CAD build for the part. Positions are in the model's coordinates, mm. Face numbers are marked on the shaded views. A direction names the side the tool comes from. Coordinates: 2 decimals unless noted, no trailing zeros. Write each loop counter-clockwise with the first axis right and the second up, starting at its lowest first coordinate (ties: lowest second). Pieces come first, ordered by that corner, then holes. Notation, with made-up numbers: (-32, 85) - (24, 85) arc R26 ccw to (24, 106) - close; hole circle Ø4 at (54, 54). An arc over 180 degrees is marked (long way). One line per question, with ' | ' between items. Start each with the question number.
1. Which spindle directions (+Z, -Z, +X, -X, +Y, -Y) get a long thin tool onto all of the face, cutting with end or side? Do the marked faces 1, 2 and 3. Say none if no direction does.
2. Band-saw the part on A-A, the plane x = 33.5. Write the cut outline in (y, z), then the cut area to 3 significant figures.
3. Flat gauge pins, fed straight in: P1, Ø1.5, axis at x = -19, z = -2, coming from the +Y side; P2, Ø4, axis at x = 31, y = 9, coming from the +Z side; P3, Ø10, axis at y = 5, z = -8.5, coming from the -X side. Where does each tip first touch, or does it go through?
4. Two-plate mould, pull along Z, no slides. Class the marked faces 4, 5, 6 and 7: +Z half, -Z half, draft (parallel to the pull), parting line (faces both ways), or undercut.
5. Band-saw the part on D-D, the plane z = 14. Write the cut outline in (x, y), then the cut area to 3 significant figures.
6. Band-saw the part on C-C, the plane x = 16. Write the cut outline in (y, z), then the cut area to 3 significant figures.
7. Band-saw the part on B-B, the plane z = 0. Write the cut outline in (x, y), then the cut area to 3 significant figures.
8. Probe line 1 (Z direction, x = 43.5, y = 13); line 2 (Y direction, x = 27.5, z = 5); line 3 (Z direction, x = 9.5, y = 9.25). List the from-to ranges inside material, lowest first.
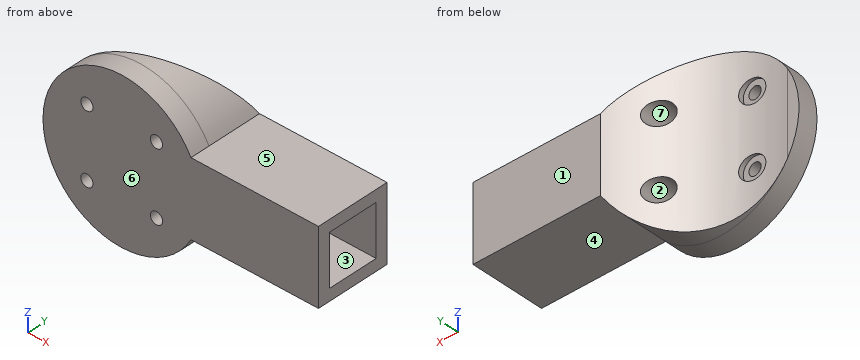
from build123d import *

# Parameters (mm, degrees)
BOSS_EXTRUDE1_DEPTH     = 2.5
SKETCH2_R               = 1.55
CUT_EXTRUDE1_DEPTH      = 2.5
SKETCH6_W               = 19
SKETCH6_H               = 19
BOSS_EXTRUDE3_DEPTH     = 32.400284093
SKETCH8_W               = 13
SKETCH8_H               = 13
CUT_EXTRUDE2_DEPTH      = 27.400284093
FILLET2_R               = 50
CUT_EXTRUDE4_REACH      = 57.642
CUT_EXTRUDE4_END_RADIUS = 50
SKETCH13_R              = 3


with BuildPart() as part:
    # Sketch1 → Boss-Extrude1 (new, symmetric)
    with BuildSketch(Plane(origin=(0, 0, 0), x_dir=(1, 0, 0), z_dir=(0, 1, 0))):
        with BuildLine():
            Line((17.599715907, 9.5), (50, 9.5))
            Line((50, 9.5), (50, -9.5))
            Line((50, -9.5), (17.599715907, -9.5))
            ThreePointArc((17.599715907, -9.5), (-20, 0), (17.599715907, 9.5))
        make_face()
    extrude(amount=BOSS_EXTRUDE1_DEPTH, both=True)

    # Sketch2 → Cut-Extrude1 (cut, symmetric)
    with BuildSketch(Plane(origin=(0, 0, 0), x_dir=(1, 0, 0), z_dir=(0, 1, 0))):
        with Locations(Location((8.838834765, 8.838834765, 0), (0, 0, 270))):
            Circle(SKETCH2_R)
        with Locations(Location((-8.838834765, 8.838834765, 0), (0, 0, 270))):
            Circle(SKETCH2_R)
        with Locations(Location((-8.838834765, -8.838834765, 0), (0, 0, 270))):
            Circle(SKETCH2_R)
        with Locations(Location((8.838834765, -8.838834765, 0), (0, 0, 270))):
            Circle(SKETCH2_R)
    extrude(amount=CUT_EXTRUDE1_DEPTH, both=True, mode=Mode.SUBTRACT)

    # Sketch6 → Boss-Extrude3 (add)
    with BuildSketch(Plane(origin=(50, 0, 0), x_dir=(0, 0, -1), z_dir=(1, 0, 0))):
        with Locations((0, 7)):
            Rectangle(SKETCH6_W, SKETCH6_H)
    extrude(amount=-BOSS_EXTRUDE3_DEPTH)

    # Sketch8 → Cut-Extrude2 (cut)
    with BuildSketch(Plane(origin=(50, 0, 0), x_dir=(0, 0, -1), z_dir=(1, 0, 0))):
        with Locations((0, 7)):
            Rectangle(SKETCH8_W, SKETCH8_H)
    extrude(amount=-CUT_EXTRUDE2_DEPTH, mode=Mode.SUBTRACT)

    # Fillet2
    # the kernel refuses this fillet: 50 mm, written as the material it adds along each edge
    with BuildSketch(Plane(origin=(17.599715907, 2.5, -96.246757864), x_dir=(-1, 0, 0), z_dir=(0, 0, 1))) as fillet2_piece_1_section:
        with BuildLine():
            CenterArc((34.698703146, -50), FILLET2_R, 90, 43.945519562)
            Line((0, -14), (0, 0))
            Line((0, 0), (34.698703146, 0))
        make_face()
    fillet2_piece_1 = extrude(amount=192.493515729, mode=Mode.PRIVATE)
    fillet2_piece_1 = fillet2_piece_1 & Plane(origin=(0, 2.5, 0), x_dir=(0.8799857953399021, 0, 0.47500000000000003), z_dir=(0, 1, 0)) * Cylinder(20, 524, mode=Mode.PRIVATE)
    fillet2_piece_1 = fillet2_piece_1 - Plane(origin=(8.838834765, 2.5, 8.838834765), x_dir=(0, 0, 1), z_dir=(0, 1, 0)) * Cylinder(1.55, 524, mode=Mode.PRIVATE)
    fillet2_piece_1 = fillet2_piece_1 - Plane(origin=(-8.838834765, 2.5, 8.838834765), x_dir=(0, 0, 1), z_dir=(0, 1, 0)) * Cylinder(1.55, 524, mode=Mode.PRIVATE)
    fillet2_piece_1 = fillet2_piece_1 - Plane(origin=(8.838834765, 2.5, -8.838834765), x_dir=(0, 0, 1), z_dir=(0, 1, 0)) * Cylinder(1.55, 524, mode=Mode.PRIVATE)
    fillet2_piece_1 = fillet2_piece_1 - Plane(origin=(-8.838834765, 2.5, -8.838834765), x_dir=(0, 0, 1), z_dir=(0, 1, 0)) * Cylinder(1.55, 524, mode=Mode.PRIVATE)
    add(fillet2_piece_1)

    # Cut-Extrude4: up to this cylinder (the profile starts outside it)
    cut_extrude4_end = Plane(origin=(-17.098987239, 52.5, 0), z_dir=(0, 0, -1)) * Cylinder(CUT_EXTRUDE4_END_RADIUS, 233.96167, mode=Mode.PRIVATE)
    # Sketch13 → Cut-Extrude4 (cut, up to the surface)
    with BuildSketch(Plane(origin=(0, 2.5, 0), x_dir=(1, 0, 0), z_dir=(0, 1, 0)), mode=Mode.PRIVATE) as cut_extrude4_sk1:
        with Locations(Location((-8.838834765, 8.838834765, 0), (0, 0, 90))):
            Circle(SKETCH13_R)
    cut_extrude4_tool1 = extrude(cut_extrude4_sk1.sketch, amount=CUT_EXTRUDE4_REACH, mode=Mode.PRIVATE) - cut_extrude4_end
    add(cut_extrude4_tool1.solids().sort_by_distance((-8.838835, 2.5, -8.838835))[0], mode=Mode.SUBTRACT)
    # Sketch13 → Cut-Extrude4 (cut, up to the surface)
    with BuildSketch(Plane(origin=(0, 2.5, 0), x_dir=(1, 0, 0), z_dir=(0, 1, 0)), mode=Mode.PRIVATE) as cut_extrude4_sk2:
        with Locations(Location((8.838834765, 8.838834765, 0), (0, 0, 90))):
            Circle(SKETCH13_R)
    cut_extrude4_tool2 = extrude(cut_extrude4_sk2.sketch, amount=CUT_EXTRUDE4_REACH, mode=Mode.PRIVATE) - cut_extrude4_end
    add(cut_extrude4_tool2.solids().sort_by_distance((8.838835, 2.5, -8.838835))[0], mode=Mode.SUBTRACT)
    # Sketch13 → Cut-Extrude4 (cut, up to the surface)
    with BuildSketch(Plane(origin=(0, 2.5, 0), x_dir=(1, 0, 0), z_dir=(0, 1, 0)), mode=Mode.PRIVATE) as cut_extrude4_sk3:
        with Locations(Location((-8.838834765, -8.838834765, 0), (0, 0, 90))):
            Circle(SKETCH13_R)
    cut_extrude4_tool3 = extrude(cut_extrude4_sk3.sketch, amount=CUT_EXTRUDE4_REACH, mode=Mode.PRIVATE) - cut_extrude4_end
    add(cut_extrude4_tool3.solids().sort_by_distance((-8.838835, 2.5, 8.838835))[0], mode=Mode.SUBTRACT)
    # Sketch13 → Cut-Extrude4 (cut, up to the surface)
    with BuildSketch(Plane(origin=(0, 2.5, 0), x_dir=(1, 0, 0), z_dir=(0, 1, 0)), mode=Mode.PRIVATE) as cut_extrude4_sk4:
        with Locations(Location((8.838834765, -8.838834765, 0), (0, 0, 90))):
            Circle(SKETCH13_R)
    cut_extrude4_tool4 = extrude(cut_extrude4_sk4.sketch, amount=CUT_EXTRUDE4_REACH, mode=Mode.PRIVATE) - cut_extrude4_end
    add(cut_extrude4_tool4.solids().sort_by_distance((8.838835, 2.5, 8.838835))[0], mode=Mode.SUBTRACT)


solid = part.part
Filled in:
1) face 1: +Z, -Z, +X, -X, +Y | face 2: +Y | face 3: +X
2) outline: (-2.5, -9.5) - (16.5, -9.5) - (16.5, 9.5) - (-2.5, 9.5) - close; hole (0.5, -6.5) - (13.5, -6.5) - (13.5, 6.5) - (0.5, 6.5) - close | area: 192 mm²
3) P1: stops at y = 2.5 | P2: stops at z = 9.5 | P3: stops at x = -19.56
4) face 4: -Z half | face 5: +Z half | face 6: draft | face 7: undercut
5) outline: (-14.28, -2.5) - (14.28, -2.5) - (14.28, 13.57) arc R50 cw to (-14.28, 2.58) - close | area: 253 mm²
6) outline: (-2.5, -12) - (15.02, -12) - (15.02, 12) - (-2.5, 12) - close | area: 421 mm²
7) outline: (-20, -2.5) - (50, -2.5) - (50, 0.5) - (22.6, 0.5) - (22.6, 13.5) - (50, 13.5) - (50, 16.5) - (17.6, 16.5) arc R50 cw to (-17.1, 2.5) - (-20, 2.5) - close | area: 599 mm²
8) line 1: z = -9.5 to -6.5, 6.5 to 9.5 | line 2: y = -2.5 to 0.5, 13.5 to 16.5 | line 3: z = -17.6 to -11.77, -5.91 to 5.91, 11.77 to 17.6
